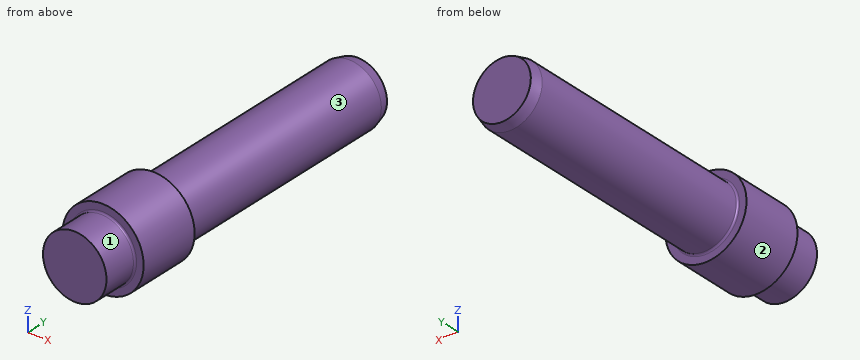
```python
from build123d import *

# Parameters (mm, degrees)
F2_R = 0.79375
F3_R = 0.79375


with BuildPart() as f1:
    # F0 (on Right) → F1 (revolve)
    with BuildSketch(Plane.YZ):
        Polygon((-15.875, 14.2875), (-15.875, 0), (142.875, 0), (142.875, 13.011392), (138.1125, 14.2875), (28.575, 14.2875), (28.575, 18.25625), (0, 18.25625), (0, 14.2875), align=None)
    revolve(axis=Axis((0, 63.5, 0), (0, 1, 0)))

    # F2
    f2_edges = [f1.edges().sort_by_distance(p)[0] for p in [
        (0, 0, -14.2875),
    ]]
    fillet(f2_edges, radius=F2_R)

    # F3
    f3_edges = [f1.edges().sort_by_distance(p)[0] for p in [
        (0, 28.575, -14.2875),
    ]]
    fillet(f3_edges, radius=F3_R)


solid = f1.part
```
The listing builds one solid part. Answer for the finished solid, in the listing's coordinates (mm). Face numbers are marked on the shaded views. A direction names the side the tool comes from. Round coordinates to 2 decimals unless told otherwise and drop trailing zeros. Loops run counter-clockwise (first coordinate to the right, second up) from the corner with the lowest first, then second, coordinate; pieces in that order, holes last.
1) A cutting plane is placed at B-B on z = 0. Determine the outline of the cut face in (x, y) (1 decimal), plus the area to 3 significant figures.
Outcome:
outline: (-18.3, 0) - (-15.1, 0) arc R0.8 cw to (-14.3, -0.8) - (-14.3, -15.9) - (14.3, -15.9) - (14.3, -0.8) arc R0.8 cw to (15.1, 0) - (18.3, 0) - (18.3, 28.6) - (15.1, 28.6) arc R0.8 cw to (14.3, 29.4) - (14.3, 138.1) - (13, 142.9) - (-13, 142.9) - (-14.3, 138.1) - (-14.3, 29.4) arc R0.8 cw to (-15.1, 28.6) - (-18.3, 28.6) - close
area: 4,760 mm2
2) A cutting plane is placed at D-D on y = 24. Determine the outline of the cut face in (x, z).
Outcome:
outline: circle Ø36.51 at (0, 0)
3) Consider line 1 (Y direction, x = -11, z = -10.5) (3 decimals); line 2 (X direction, y = 119, z = 1.5); line 3 (Z direction, x = 6.5, y = 16.5). Determine where each line is inside the solid, lowest interval first.
Outcome:
line 1: y = 0 to 28.575
line 2: x = -14.21 to 14.21
line 3: z = -17.06 to 17.06
4) For the marked faces 1, 2 and 3, determine the directions among +Z, -Z, +X, -X, +Y, -Y from which every point of the face is accessible in a straight line to the end or side of a thin tool.
Outcome:
face 1: -Y
face 2: +Y, -Y
face 3: +Y
5) A cutting plane is placed at A-A on x = 0. Determine the outline of the cut face in (y, z) (1 decimal).
Outcome:
outline: (-15.9, -14.3) - (-0.8, -14.3) arc R0.8 cw to (0, -15.1) - (0, -18.3) - (28.6, -18.3) - (28.6, -15.1) arc R0.8 cw to (29.4, -14.3) - (138.1, -14.3) - (142.9, -13) - (142.9, 13) - (138.1, 14.3) - (29.4, 14.3) arc R0.8 cw to (28.6, 15.1) - (28.6, 18.3) - (0, 18.3) - (0, 15.1) arc R0.8 cw to (-0.8, 14.3) - (-15.9, 14.3) - close
6) A cutting plane is placed at C-C on y = 108. Determine the outline of the cut face in (x, z) (1 decimal), plus the area to 3 significant figures.
Outcome:
outline: circle Ø28.6 at (0, 0)
area: 641 mm2
7) Given P1, Ø8, axis at x = -11.5, y = 66, coming from the -Z side; P2, Ø2, axis at x = 7, y = 61, coming from the -Z side; P3, Ø1.5, axis at y = 4.5, z = -13.5, coming from the -X side, each flat-ended and moving along its own axis, determine where each tip first touches the part or whether it passes through.
Outcome:
P1: stops at z = -12.16
P2: stops at z = -12.97
P3: stops at x = -13.07
